Geometry: see drawing. Coordinates: mm, zero at the bounding-box minimum. A direction names the side the tool comes from. Give positions to 0.01 mm unless a question says otherwise; leave off trailing zeros. Loops run counter-clockwise (first coordinate to the right, second up) from the corner with the lowest first, then second, coordinate; pieces in that order, holes last. Notation, with made-up numbers: (-24, 82) - (11, 82) arc R23 cw to (11, 109) - close; hole circle Ø6 at (42, 19). An arc over 180 degrees is marked (long way). Use one line per item in the form item = value.
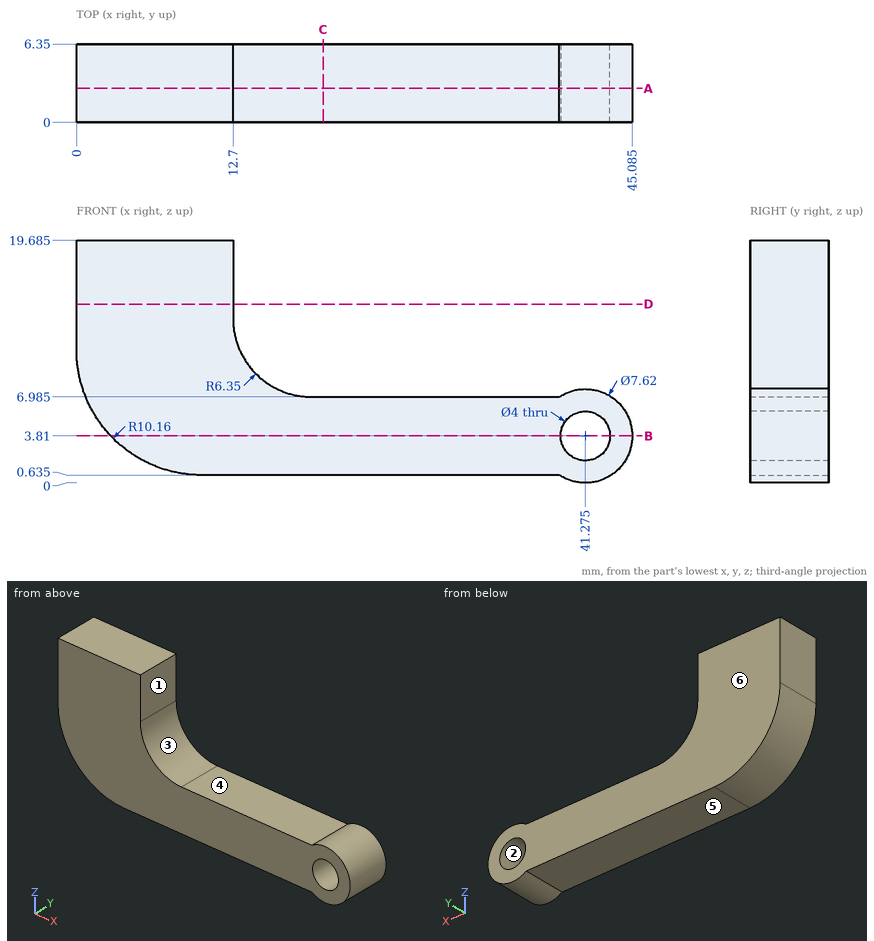
(1) Cut plane B-B (z = 3.81). Return the cut outline in (x, y) (3 decimals), plus the area to 3 significant figures.
Solution:
outline = (2.782, 0) - (39.275, 0) - (39.275, 6.35) - (2.782, 6.35) - close; (43.275, 0) - (45.085, 0) - (45.085, 6.35) - (43.275, 6.35) - close
area = 243 mm2
(2) Cut plane D-D (z = 14.5). Return the cut outline in (x, y).
Solution:
outline = (0, 0) - (12.7, 0) - (12.7, 6.35) - (0, 6.35) - close
(3) Pull-direction query (Z, two-part tool) for the marked faces 1, 2 and 3; classes: released by +Z, released by -Z, zero draft, split by the parting line, or undercut.
Solution:
face_1 = zero draft
face_2 = undercut
face_3 = released by +Z
(4) Material intervals for L1, parallel to Z at x = 33.5, y = 1.5 (3 decimals); L2, parallel to X at y = 5.25, z = 13.25; L3, parallel to X at y = 2.75, z = 3.81 (1 decimal), sorted ascending. Write a range as from..to.
Solution:
L1 = 0.635..6.985
L2 = 0..12.7
L3 = 2.8..39.3, 43.3..45.1
(5) Cut plane C-C (x = 20). Return the cut outline in (y, z) (3 decimals).
Solution:
outline = (0, 0.635) - (6.35, 0.635) - (6.35, 6.985) - (0, 6.985) - close
(6) Pin query (flat end, axial travel): P1, Ø1.5, axis at x = 38, y = 3.5, coming from the -Z side (3 decimals); P2, Ø1.9, axis at y = 3.5, z = 16, coming from the +X side; P3, Ø1.5, axis at x = 22, y = 4, coming from the +Z side (3 decimals). Return the tip coordinate at first contact, or that it passes through.
Solution:
P1 = 0.635
P2 = 12.7
P3 = 6.985
(7) Cut plane A-A (y = 2.75). Return the cut outline in (x, z) (3 decimals).
Solution:
outline = (0, 10.795) arc R10.16 ccw to (10.16, 0.635) - (39.169, 0.635) arc R3.81 ccw (long way) to (39.169, 6.985) - (19.05, 6.985) arc R6.35 cw to (12.7, 13.335) - (12.7, 19.685) - (0, 19.685) - close; hole circle Ø4 at (41.275, 3.81)
(8) Access query for the marked faces 4, 5 and 6. Directions: +Z, -Z, +X, -X, +Y, -Y. A direction counts if a zero-diameter tool reaches every point of the face in a straight line with its end or side. Return the directions, or none.
Solution:
face_4 = +Z, +Y, -Y
face_5 = -Z, -X, +Y, -Y
face_6 = +Z, -Z, +X, -X, +Y
